from build123d import *

# Parameters (mm, degrees)
SKETCH_1_W          = 40
SKETCH_1_H          = 20
EXTRUDE_1_DEPTH     = 40.5
SKETCH_2_R          = 3
EXTRUDE_2_DEPTH     = 7
EXTRUDE_START       = -5
SKETCH_3_W          = 7
SKETCH_3_H          = 20
EXTRUDE_3_DEPTH     = 3
SKETCH_4_R          = 2.5
CUT_EXTRUDE_1_DEPTH = 10


with BuildPart() as part:
    # 草图1 → 凸台-拉伸1 (new body)
    with BuildSketch(Plane.XY):
        with Locations((20, -10)):
            Rectangle(SKETCH_1_W, SKETCH_1_H)
    extrude(amount=EXTRUDE_1_DEPTH)

    # 草图2 → 凸台-拉伸2 (add)
    with BuildSketch(Plane.XY.offset(40.5)):
        with Locations((10, -10)):
            Circle(SKETCH_2_R)
    extrude(amount=EXTRUDE_2_DEPTH)

    # 草图3 → 凸台-拉伸3 (add)
    with BuildSketch(Plane.XY.offset(40.5).offset(EXTRUDE_START)):
        with Locations((43.5, -10)):
            Rectangle(SKETCH_3_W, SKETCH_3_H)
        with Locations((-3.5, -10)):
            Rectangle(SKETCH_3_W, SKETCH_3_H)
    extrude(amount=-EXTRUDE_3_DEPTH)

    # 草图4 → 切除-拉伸1 (cut)
    with BuildSketch(Plane.XY.offset(35.5)):
        with Locations((-5, -5)):
            Circle(SKETCH_4_R)
        with Locations((45, -5)):
            Circle(SKETCH_4_R)
        with Locations((-5, -15)):
            Circle(SKETCH_4_R)
        with Locations((45, -15)):
            Circle(SKETCH_4_R)
    extrude(amount=-CUT_EXTRUDE_1_DEPTH, mode=Mode.SUBTRACT)


solid = part.part
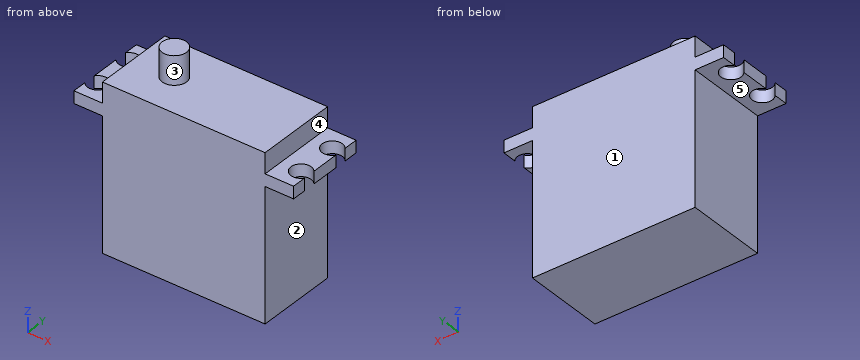
Check sheet for the modelled part. Datum: model origin and axes. Units: mm. Face numbers are marked on the shaded views. A direction names the side the tool comes from. Coordinates: 2 decimals unless noted, no trailing zeros. Loops run counter-clockwise (first coordinate to the right, second up) from the corner with the lowest first, then second, coordinate; pieces in that order, holes last. Notation, with made-up numbers: (-39, 41.5) -> (-4, 41.5) arc R15 cw to (-4, 66.5) -> close; hole circle Ø6 at (59, 20). An arc over 180 degrees is marked (long way). Write item = value, one per line. Start each with the question number.
1. Tool access check on the marked faces 1, 2, 3, 4 and 5. Record the directions out of +Z, -Z, +X, -X, +Y, -Y that give a thin tool (end or side, any length) a straight path to the whole face; none if there is none.
2. Section check A-A on x = -5. Record the cut outline in (y, z).
3. Depth check by flat-ended pin: P1, Ø2, axis at x = -2.5, y = -11.5, coming from the -Z side; P2, Ø5, axis at x = 18, y = -6, coming from the +Z side; P3, Ø2.5, axis at y = -13.5, z = 38.5, coming from the +X side; P4, Ø4.5, axis at x = 45, y = -15, coming from the +Z side. Enter the tip coordinate at first touch or a pass-through.
4. Section check C-C on x = 10. Record the cut outline in (y, z).
5. Section check B-B on y = -5. Record the cut outline in (x, z).
6. Material ranges on line 1 (Y direction, x = 45, z = 33.55); line 2 (X direction, y = -6.25, z = 5.5); line 3 (Z direction, x = 42, y = -5.5), recorded low to high.
7. Section check D-D on z = 5.5. Record the cut outline in (x, y).
Responses:
q1.face_1 = +Z, -Z, +X, -X, +Y
q1.face_2 = -Z, +X, +Y, -Y
q1.face_3 = +Z
q1.face_4 = +Z, +X, +Y, -Y
q1.face_5 = -Z, -X, +Y, -Y
q2.outline = (-20, 32.5) -> (-17.5, 32.5) -> (-17.5, 35.5) -> (-20, 35.5) -> close; (-12.5, 32.5) -> (-7.5, 32.5) -> (-7.5, 35.5) -> (-12.5, 35.5) -> close; (-2.5, 32.5) -> (0, 32.5) -> (0, 35.5) -> (-2.5, 35.5) -> close
q3.P1 = 32.5
q3.P2 = 40.5
q3.P3 = 40
q3.P4 = through
q4.outline = (-20, 0) -> (0, 0) -> (0, 40.5) -> (-7, 40.5) -> (-7, 47.5) -> (-13, 47.5) -> (-13, 40.5) -> (-20, 40.5) -> close
q5.outline = (-2.5, 32.5) -> (0, 32.5) -> (0, 0) -> (40, 0) -> (40, 32.5) -> (42.5, 32.5) -> (42.5, 35.5) -> (40, 35.5) -> (40, 40.5) -> (0, 40.5) -> (0, 35.5) -> (-2.5, 35.5) -> close
q6.line_1 = -20 to -17.5, -12.5 to -7.5, -2.5 to 0
q6.line_2 = 0 to 40
q6.line_3 = 32.5 to 35.5
q7.outline = (0, -20) -> (40, -20) -> (40, 0) -> (0, 0) -> close
